The listing builds one solid part. Answer for the finished solid, in the listing's coordinates (mm). A direction names the side the tool comes from. Give positions to 0.01 mm unless a question says otherwise; leave off trailing zeros. Write each question's results on one line, items separated by ' | '. Start each with the question number.
Q1. For a pull along X with two mould halves and no side action, classify faces 4 (the face through (0, 139, 3.655)), 5 (the face through (0, 139, -3.655)), 6 (the face through (6, 139, 10)), 7 (the face through (-10, 139, -6)) as pulls with the +X half, pulls with the -X half, needs draft (parallel to the pull), parting line crosses it, or undercut.
Q2. For faces 1 (the face through (3.655, 139, 0)), 2 (the face through (-6, 139, -10)), 3 (the face through (-3.655, 139, 0)), determine the directions among +Z, -Z, +X, -X, +Y, -Y from which every point of the face is accessible in a straight line to the end or side of a thin tool.
Q3. Flat-ended cylindrical pins translate along their axes: pin 1 Ø3.5 at (y, z) = (208.5, 0.5) entering from -X (3 decimals); pin 2 Ø1.5 at (y, z) = (36.5, -1) entering from +X (3 decimals). Find the tip coordinate at first contact, or state that the pin passes through.
Q4. Find the intervals of material crossed by probe 1 along X at (y, z) = (37.5, -3.25); probe 2 along Z at (x, y) = (4.75, 144.5); probe 3 along Z at (x, y) = (3.5, 235), in increasing order.
Autodesk Inventor part; units mm, degrees
ref_plane "YZ Plane" through (0, 0, 0) normal (1, 0, 0) x (0, 1, 0)
ref_plane "XZ Plane" through (0, 0, 0) normal (0, 1, 0) x (-1, 0, 0)
ref_plane "XY Plane" through (0, 0, 0) normal (0, 0, 1) x (1, 0, 0)
sketch "Sketch1" plane through (0, 0, 0) normal (0, 1, 0) x (-1, 0, 0)
  line L0 (0, -14) -> (0, 14)
  line L1 (-14, 0) -> (14, 0)
  line L2 (14, 0) -> (-14, 0)
  line L3 (0, -14) -> (0, 14)
  line L4 (2.5943, 3.655) -> (-2.5943, 3.655)
  line L5 (-3.655, 2.5943) -> (-3.655, -2.5943)
  line L6 (-2.5943, -3.655) -> (2.5943, -3.655)
  line L7 (3.655, -2.5943) -> (3.655, 2.5943)
  line L8 (-3.655, 3.655) -> (3.655, -3.655) construction
  line L9 (10, 10) -> (10, 2.63)
  line L10 (10, 2.63) -> (8.5, 2.63)
  line L11 (10, 10) -> (2.63, 10)
  line L12 (2.63, 10) -> (2.63, 8.5)
  line L13 (-10, 10) -> (-2.63, 10)
  line L14 (-2.63, 10) -> (-2.63, 8.5)
  line L15 (-10, 8.5) -> (-10, 10)
  line L16 (-10, 10) -> (-8.5, 10)
  line L17 (-8.5, 2.63) -> (-10, 2.63)
  line L18 (-10, 2.63) -> (-10, 10)
  line L19 (-10, -10) -> (-8.5, -10)
  line L20 (-8.5, -2.63) -> (-10, -2.63)
  line L21 (-10, -2.63) -> (-10, -10)
  line L22 (-10, -10) -> (-2.63, -10)
  line L23 (-2.63, -10) -> (-2.63, -8.5)
  line L24 (-10, -8.5) -> (-10, -10)
  line L25 (10, -10) -> (8.5, -10)
  line L26 (8.5, -2.63) -> (10, -2.63)
  line L27 (10, -2.63) -> (10, -10)
  line L28 (10, -10) -> (2.63, -10)
  line L29 (2.63, -10) -> (2.63, -8.5)
  line L30 (10, -8.5) -> (10, -10)
  circle A0 centre (0, 0) radius 2.095
  line L31 (5.995, -10) -> (2.63, -10)
  line L32 (-2.63, -10) -> (-5.995, -10)
  line L33 (10, -10) -> (2.63, -10)
  line L34 (-2.63, -10) -> (-10, -10)
  line L35 (10, -5.995) -> (10, -2.63)
  line L36 (10, 2.63) -> (10, 5.995)
  line L37 (10, 10) -> (10, 2.63)
  line L38 (10, -2.63) -> (10, -10)
  line L39 (-5.995, 10) -> (-2.63, 10)
  line L40 (2.63, 10) -> (5.995, 10)
  line L41 (-10, 10) -> (-2.63, 10)
  line L42 (2.63, 10) -> (10, 10)
  line L43 (-10, 5.995) -> (-10, 2.63)
  line L44 (-10, -2.63) -> (-10, -5.995)
  line L45 (-10, -10) -> (-10, -2.63)
  line L46 (-10, 2.63) -> (-10, 10)
  line L47 (-2.63, -8.5) -> (-5.995, -8.5)
  line L48 (-8.5, -5.995) -> (-8.5, -2.63)
  line L49 (-8.5, -5.995) -> (-7.0557, -5.995)
  line L50 (-5.995, -8.5) -> (-5.995, -7.0557)
  line L51 (-5.995, 7.0557) -> (-5.995, 8.5)
  line L52 (2.63, 8.5) -> (5.995, 8.5)
  line L53 (8.5, 2.63) -> (8.5, 5.995)
  line L54 (8.5, 5.995) -> (7.0557, 5.995)
  line L55 (5.995, 8.5) -> (5.995, 7.0557)
  line L56 (2.63, -8.5) -> (5.995, -8.5)
  line L57 (9.5607, -8.5) -> (10, -8.5)
  line L58 (8.5, -10) -> (8.5, -9.5607)
  line L59 (8.5, -5.995) -> (8.5, -2.63)
  line L60 (7.0557, -5.995) -> (8.5, -5.995)
  line L61 (5.995, -7.0557) -> (5.995, -8.5)
  line L62 (3.655, 3.655) -> (-0.5303, -0.5303) construction
  line L63 (-1.4814, -1.4814) -> (-3.655, -3.655) construction
  line L64 (-8.5, 10) -> (-8.5, 9.5607)
  line L65 (-8.5, 5.995) -> (-8.5, 2.63)
  line L66 (-2.63, 8.5) -> (-5.995, 8.5)
  line L67 (-9.5607, 8.5) -> (-10, 8.5)
  line L68 (-7.0557, 5.995) -> (-8.5, 5.995)
  line L69 (-3.655, 2.5943) -> (-7.0557, 5.995)
  line L70 (-2.5943, 3.655) -> (-5.995, 7.0557)
  line L71 (5.995, 7.0557) -> (2.5943, 3.655)
  line L72 (7.0557, 5.995) -> (3.655, 2.5943)
  line L73 (7.0557, -5.995) -> (3.655, -2.5943)
  line L74 (5.995, -7.0557) -> (2.5943, -3.655)
  line L75 (-2.5943, -3.655) -> (-5.995, -7.0557)
  line L76 (-3.655, -2.5943) -> (-7.0557, -5.995)
  dimension "d26" = 4.19
  dimension "d0" = 20
  dimension "d1" = 20
  dimension "d2" = 7.31
  dimension "d3" = 7.31
  dimension "d4" = 20
  dimension "d5" = 11.99
  dimension "d6" = 11.99
  dimension "d11" = 7.37
  dimension "d12" = 1.5
  dimension "d13" = 7.37
  dimension "d14" = 1.5
  dimension "d15" = 7.37
  dimension "d16" = 1.5
  dimension "d17" = 7.37
  dimension "d18" = 1.5
  dimension "d19" = 7.37
  dimension "d20" = 7.37
  dimension "d21" = 1.5
  dimension "d22" = 1.5
  dimension "d23" = 7.37
  dimension "d24" = 7.37
  dimension "d25" = 1.5
extrude "Extrusion1" add sketch "Sketch1" along normal blind 282.2194 contours L6 L75 L50 L47 L23 L22 L19 L21 L20 L48 L49 L76 L5 L1 A0 L0 | L0 A0 L1 L7 L73 L60 L59 L26 L27 L25 L28 L29 L56 L61 L74 L6 | L1 L5 L69 L68 L65 L17 L18 L15 L13 L14 L66 L51 L70 L4 L0 A0 | A0 L0 L4 L71 L55 L52 L12 L11 L9 L10 L53 L54 L72 L7 L1
fillet "Fillet1" radius 0.5 20 edges at (10, 141.1097, 10) (2.63, 141.1097, 10) (-2.63, 141.1097, 10) (-2.63, 141.1097, 8.5) (10, 141.1097, 2.63) (8.5, 141.1097, 2.63) (10, 141.1097, -2.63) (8.5, 141.1097, -2.63) (10, 141.1097, -10) (2.63, 141.1097, -8.5) (-2.63, 141.1097, -10) (-2.63, 141.1097, -8.5) (2.63, 141.1097, -10) (-10, 141.1097, -10) (-8.5, 141.1097, -2.63) (-10, 141.1097, -2.63) (-8.5, 141.1097, 2.63) (-10, 141.1097, 2.63) (-10, 141.1097, 10) (2.63, 141.1097, 8.5)
fillet "Fillet2" radius 0.75 24 edges at (-7.0557, 141.1097, 5.995) (-3.655, 141.1097, 2.5943) (-8.5, 141.1097, -5.995) (-7.0557, 141.1097, -5.995) (-5.995, 141.1097, -8.5) (3.655, 141.1097, -2.5943) (7.0557, 141.1097, -5.995) (-2.5943, 141.1097, 3.655) (-5.995, 141.1097, 7.0557) (3.655, 141.1097, 2.5943) (7.0557, 141.1097, 5.995) (8.5, 141.1097, 5.995) (8.5, 141.1097, -5.995) (2.5943, 141.1097, 3.655) (5.995, 141.1097, 7.0557) (5.995, 141.1097, 8.5) (-5.995, 141.1097, 8.5) (-8.5, 141.1097, 5.995) (2.5943, 141.1097, -3.655) (5.995, 141.1097, -7.0557) (5.995, 141.1097, -8.5) (-5.995, 141.1097, -7.0557) (-2.5943, 141.1097, -3.655) (-3.655, 141.1097, -2.5943)
properties part number "proWildStangin"
Answers below:
1) face 4: undercut | face 5: undercut | face 6: needs draft | face 7: pulls with the -X half
2) face 1: +X, +Y, -Y | face 2: -Z, +X, -X, +Y, -Y | face 3: -X, +Y, -Y
3) pin 1: stops at x = -3.655 | pin 2: stops at x = 3.655
4) probe 1: x = -10 to -8.5, -4.31 to 4.31, 8.5 to 10 | probe 2: z = -10 to -8.5, -5.81 to -3.69, 3.69 to 5.81, 8.5 to 10 | probe 3: z = -10 to -8.5, -4.56 to 4.56, 8.5 to 10
